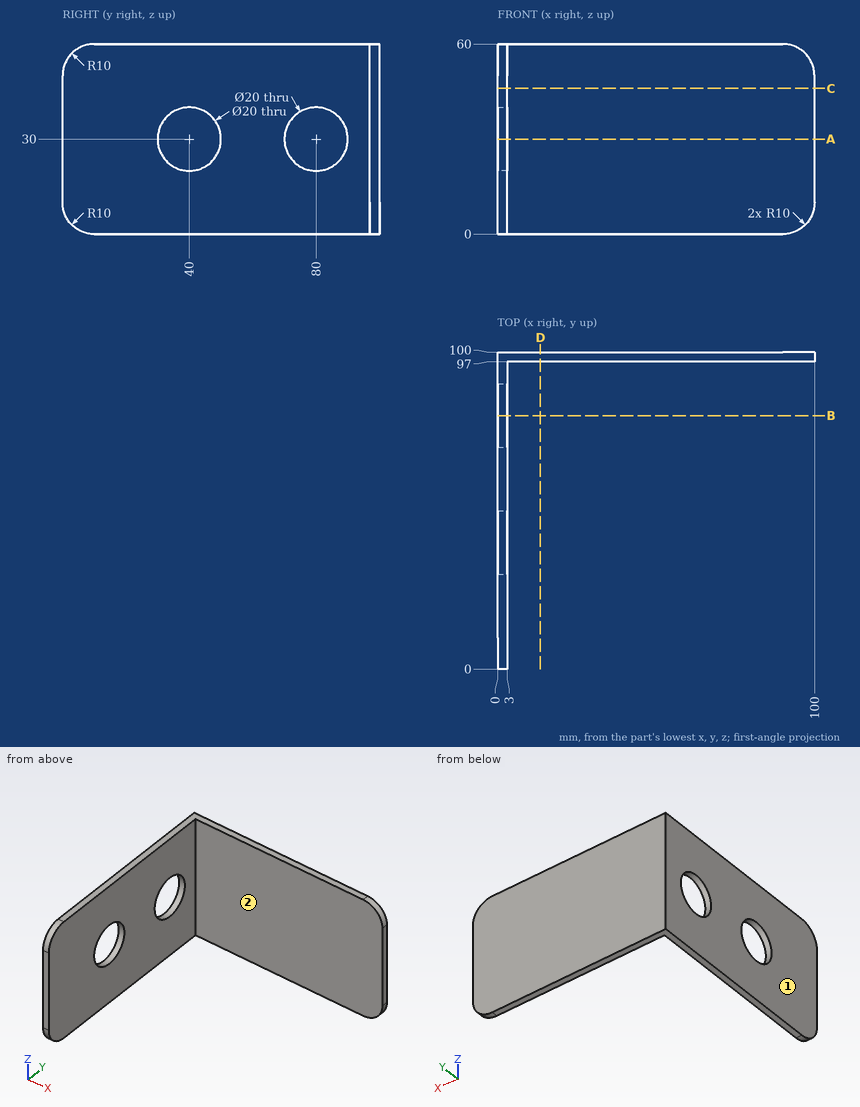
Geometry check sheet. Reference: drawing and pictorial views, mm from the part's lowest x, y, z. A direction names the side the tool comes from. Coordinates: 2 decimals unless noted, no trailing zeros. Order: outer loops, then holes, each group sorted by start corner. A loop starts at its lowest first (then second) coordinate and runs counter-clockwise, first axis right, second up.
Item 1: Section check A-A, the plane z = 30. Enter the section's corners in (x, y), then the cut area to 3 significant figures.
Filled in:
outline: (0, 0) - (3, 0) - (3, 30) - (0, 30) - close; (0, 50) - (3, 50) - (3, 70) - (0, 70) - close; (0, 90) - (3, 90) - (3, 97) - (100, 97) - (100, 100) - (0, 100) - close
area: 471 mm2
Item 2: Section check C-C, the plane z = 46. Enter the section's corners in (x, y), then the cut area to 3 significant figures.
Filled in:
outline: (0, 0) - (3, 0) - (3, 97) - (100, 97) - (100, 100) - (0, 100) - close
area: 591 mm2
Item 3: Access from +Z, -Z, +X, -X, +Y, -Y to the whole of each face (thin tool, end or side, straight path). Record for the marked faces 1 and 2.
Filled in:
face 1: +Z, -Z, -X, +Y, -Y
face 2: +Z, -Z, +X, -Y
Item 4: Material ranges on L1, parallel to Y at x = 2, z = 30; L2, parallel to X at y = 20.5, z = 16.5; L3, parallel to Y at x = 76, z = 49, recorded low to high.
Filled in:
L1: y = 0 to 30, 50 to 70, 90 to 100
L2: x = 0 to 3
L3: y = 97 to 100
Item 5: Section check B-B, the plane y = 80. Enter the section's corners in (x, z).
Filled in:
outline: (0, 0) - (3, 0) - (3, 20) - (0, 20) - close; (0, 40) - (3, 40) - (3, 60) - (0, 60) - close
Item 6: Depth check by flat-ended pin: pin 1 (6 mm diameter, centred on x = 36, z = 19, fed in from -Y); pin 2 (5 mm diameter, centred on y = 87.5, z = 50, fed in from -X); pin 3 (12 mm diameter, centred on y = 40, z = 30, fed in from -X); pin 4 (18 mm diameter, centred on y = 67, z = 31, fed in from +X). Enter the tip coordinate at first touch or a pass-through.
Filled in:
pin 1: stops at y = 97
pin 2: stops at x = 0
pin 3: passes through
pin 4: stops at x = 3
Item 7: Section check D-D, the plane x = 13.5. Enter the section's corners in (y, z), then the cut area to 3 significant figures.
Filled in:
outline: (97, 0) - (100, 0) - (100, 60) - (97, 60) - close
area: 180 mm2
